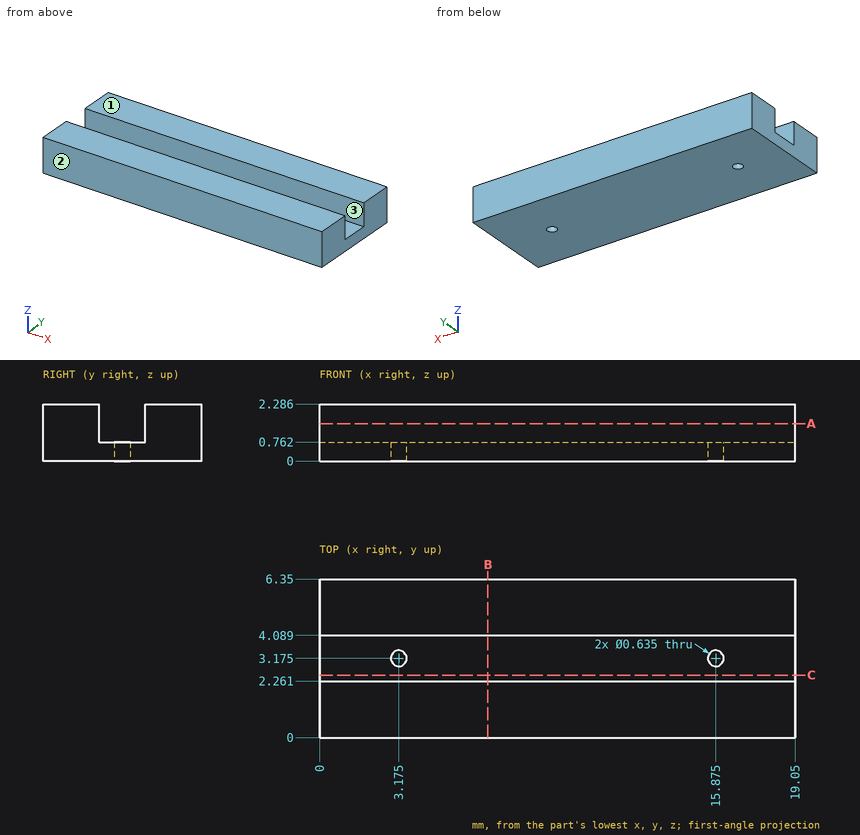
Print and shaded views of the part. All mm, measured from the part's lowest x, y and z. Coordinates: 2 decimals unless noted, no trailing zeros. Order: outer loops, then holes, each group sorted by start corner. A loop starts at its lowest first (then second) coordinate and runs counter-clockwise, first axis right, second up. Notation, with made-up numbers: (18.5, 82.25) -> (44.5, 82.25) arc R10 cw to (44.5, 101.25) -> close; hole circle Ø3 at (-24, 36). An arc over 180 degrees is marked (long way). Answer as a JSON object with one key per item and string values. Group by question number.
1) Drill centre lines: L1, parallel to Y at x = 1.75, z = 1.4; L2, parallel to Z at x = 13.25, y = 2.75; L3, parallel to Y at x = 16, z = 0.65. Where is each one in solid material? Low to high.
2) Flat gauge pin, fed straight in: pin 1 (0.9 mm diameter, centred on x = 14, y = 3.5, fed in from +Z). Where does the tip first touch, or does it go through?
3) Pull direction Y, two halves, no side cores. Call the marked faces 1, 2 and 3: +Y half, -Y half, draft (parallel to the pull), parting line (faces both ways), or undercut.
4) Cut at A-A, the plane z = 1.5. Write the cut outline in (x, y).
5) Cut at C-C, the plane y = 2.5. Write the cut outline in (x, z), then the cut area to 3 significant figures.
6) Cut at B-B, the plane x = 6.75. Write the cut outline in (y, z), then the cut area to 3 significant figures.
Check values:
{
 "1": {"L1": "y = 0 to 2.26, 4.09 to 6.35", "L2": "z = 0 to 0.76", "L3": "y = 0 to 2.88, 3.47 to 6.35"},
 "2": {"pin 1": "stops at z = 0.76"},
 "3": {"face 1": "draft", "face 2": "-Y half", "face 3": "undercut"},
 "4": {"outline": "(0, 0) -> (19.05, 0) -> (19.05, 2.26) -> (0, 2.26) -> close; (0, 4.09) -> (19.05, 4.09) -> (19.05, 6.35) -> (0, 6.35) -> close"},
 "5": {"outline": "(0, 0) -> (19.05, 0) -> (19.05, 0.76) -> (0, 0.76) -> close", "area": "14.5 mm²"},
 "6": {"outline": "(0, 0) -> (6.35, 0) -> (6.35, 2.29) -> (4.09, 2.29) -> (4.09, 0.76) -> (2.26, 0.76) -> (2.26, 2.29) -> (0, 2.29) -> close", "area": "11.7 mm²"}
}
